from build123d import *

# Parameters (mm, degrees)
ESBO_O1_W                = 5
ESBO_O1_H                = 4.65
RESSALTO_EXTRUS_O1_DEPTH = 120
RESSALTO_EXTRUS_O2_DEPTH = 4.75
F_3_0MM_DOWEL_HOLE3_D    = 3
CUT_EXTRUDE2_DEPTH       = 10
FILLET4_START            = -3
FILLET4_DEPTH            = 6
FILLET1_SIZE             = 0.5
FILLET6_START            = -2.325
FILLET6_DEPTH            = 4.65
FILLET7_START            = -2.325
FILLET7_DEPTH            = 4.65


with BuildPart() as part:
    # Esboço1 → Ressalto-extrusão1 (new body)
    with BuildSketch(Plane(origin=(0, 0, 0), x_dir=(0, 0, -1), z_dir=(1, 0, 0))):
        with Locations((-2.5, 0)):
            Rectangle(ESBO_O1_W, ESBO_O1_H)
    extrude(amount=RESSALTO_EXTRUS_O1_DEPTH)

    # Esboço2 → Ressalto-extrusão2 (add)
    with BuildSketch(Plane(origin=(0, 2.325, 0), x_dir=(1, 0, 0), z_dir=(0, 1, 0))):
        Polygon((75, 0), (87.5, 0), (86.75, 4.5), align=None)
    extrude(amount=-RESSALTO_EXTRUS_O2_DEPTH)

    # Ø3.0mm Dowel Hole3 (through all)
    with Locations(Plane(origin=(0, 0, 0), x_dir=(-1, 0, 0), z_dir=(0, 0, -1))):
        with Locations((-5, 0), (-10, 0), (-15, 0), (-20, 0)):
            Hole(F_3_0MM_DOWEL_HOLE3_D / 2)

    # Sketch12 → Cut-Extrude2 (cut)
    with BuildSketch(Plane(origin=(0, 2.325, 0), x_dir=(1, 0, 0), z_dir=(0, 1, 0))):
        with BuildLine():
            Line((120, -2.5), (108.780523662, -2.5))
            ThreePointArc((108.780523662, -2.5), (105.971779801, -1.840547319), (103.75, 0))
            Line((103.75, 0), (120, 0))
            Line((120, 0), (120, -2.5))
        make_face()
    extrude(amount=-CUT_EXTRUDE2_DEPTH, mode=Mode.SUBTRACT)

    # Fillet4: read off the stored shape, not the designer's step
    # Fillet4 outline → Fillet4 (cut)
    with BuildSketch(Plane(origin=(0, 0, 0), x_dir=(1, 0, 0), z_dir=(0, 1, 0)).offset(FILLET4_START)):
        with BuildLine():
            add(Edge.make_bspline(
                [(104.477311177, -0.805478659), (103.613151376, 0), (102.431809752, 0)],
                knots=[0, 0, 0, 1, 1, 1], degree=2, weights=[1, 2.791376365, 1]))
            ThreePointArc((104.477311177, -0.805478659), (104.096310112, -0.418401518), (103.75, 0))
            Line((103.75, 0), (102.431809752, 0))
        make_face()
        with BuildLine():
            Line((120, -2.5), (117.041960108, -2.5))
            add(Edge.make_bspline(
                [(120, -5), (119.577422873, -2.5), (117.041960108, -2.5)],
                knots=[0, 0, 0, 1, 1, 1], degree=2, weights=[1, 2.291287847, 1]))
            Line((120, -5), (120, -2.5))
        make_face()
    extrude(amount=FILLET4_DEPTH, mode=Mode.SUBTRACT)

    # Fillet1
    # a fillet whose section is not a circle: 0.5 mm, written as the material it takes off along each edge
    with BuildSketch(Plane(origin=(20, 0, 0), x_dir=(1, 0, 0), z_dir=(0, -1, 0))) as fillet1_piece_1:
        with BuildLine():
            Bezier((1.5 + FILLET1_SIZE, 0), (1.5, 0), (1.5, FILLET1_SIZE), weights=[1, 0.353553391, 1])
            Line((1.5, FILLET1_SIZE), (1.5 - FILLET1_SIZE * 0.02, FILLET1_SIZE))
            Line((1.5 - FILLET1_SIZE * 0.02, FILLET1_SIZE), (1.5 - FILLET1_SIZE * 0.02, -FILLET1_SIZE * 0.02))
            Line((1.5 - FILLET1_SIZE * 0.02, -FILLET1_SIZE * 0.02), (1.5 + FILLET1_SIZE, -FILLET1_SIZE * 0.02))
            Line((1.5 + FILLET1_SIZE, -FILLET1_SIZE * 0.02), (1.5 + FILLET1_SIZE, 0))
        make_face()
    revolve(axis=Axis((20, 0, 0), (0, 0, 1)), mode=Mode.SUBTRACT)
    with BuildSketch(Plane(origin=(15, 0, 0), x_dir=(1, 0, 0), z_dir=(0, -1, 0))) as fillet1_piece_2:
        with BuildLine():
            Bezier((1.5 + FILLET1_SIZE, 0), (1.5, 0), (1.5, FILLET1_SIZE), weights=[1, 0.353553391, 1])
            Line((1.5, FILLET1_SIZE), (1.5 - FILLET1_SIZE * 0.02, FILLET1_SIZE))
            Line((1.5 - FILLET1_SIZE * 0.02, FILLET1_SIZE), (1.5 - FILLET1_SIZE * 0.02, -FILLET1_SIZE * 0.02))
            Line((1.5 - FILLET1_SIZE * 0.02, -FILLET1_SIZE * 0.02), (1.5 + FILLET1_SIZE, -FILLET1_SIZE * 0.02))
            Line((1.5 + FILLET1_SIZE, -FILLET1_SIZE * 0.02), (1.5 + FILLET1_SIZE, 0))
        make_face()
    revolve(axis=Axis((15, 0, 0), (0, 0, 1)), mode=Mode.SUBTRACT)
    with BuildSketch(Plane(origin=(10, 0, 0), x_dir=(1, 0, 0), z_dir=(0, -1, 0))) as fillet1_piece_3:
        with BuildLine():
            Bezier((1.5 + FILLET1_SIZE, 0), (1.5, 0), (1.5, FILLET1_SIZE), weights=[1, 0.353553391, 1])
            Line((1.5, FILLET1_SIZE), (1.5 - FILLET1_SIZE * 0.02, FILLET1_SIZE))
            Line((1.5 - FILLET1_SIZE * 0.02, FILLET1_SIZE), (1.5 - FILLET1_SIZE * 0.02, -FILLET1_SIZE * 0.02))
            Line((1.5 - FILLET1_SIZE * 0.02, -FILLET1_SIZE * 0.02), (1.5 + FILLET1_SIZE, -FILLET1_SIZE * 0.02))
            Line((1.5 + FILLET1_SIZE, -FILLET1_SIZE * 0.02), (1.5 + FILLET1_SIZE, 0))
        make_face()
    revolve(axis=Axis((10, 0, 0), (0, 0, 1)), mode=Mode.SUBTRACT)
    with BuildSketch(Plane(origin=(5, 0, 0), x_dir=(1, 0, 0), z_dir=(0, -1, 0))) as fillet1_piece_4:
        with BuildLine():
            Bezier((1.5 + FILLET1_SIZE, 0), (1.5, 0), (1.5, FILLET1_SIZE), weights=[1, 0.353553391, 1])
            Line((1.5, FILLET1_SIZE), (1.5 - FILLET1_SIZE * 0.02, FILLET1_SIZE))
            Line((1.5 - FILLET1_SIZE * 0.02, FILLET1_SIZE), (1.5 - FILLET1_SIZE * 0.02, -FILLET1_SIZE * 0.02))
            Line((1.5 - FILLET1_SIZE * 0.02, -FILLET1_SIZE * 0.02), (1.5 + FILLET1_SIZE, -FILLET1_SIZE * 0.02))
            Line((1.5 + FILLET1_SIZE, -FILLET1_SIZE * 0.02), (1.5 + FILLET1_SIZE, 0))
        make_face()
    revolve(axis=Axis((5, 0, 0), (0, 0, 1)), mode=Mode.SUBTRACT)

    # Fillet5
    # a fillet whose section is not a circle: 2 mm, written as the material it takes off along each edge
    with BuildSketch(Plane(origin=(86.75, 8.443980956, -4.5), x_dir=(-0.9338567516961642, 0, 0.35764726660704255), z_dir=(0, -1, 0))) as fillet5_piece_1:
        with BuildLine():
            Bezier((2.447592383, 0), (0, 0), (0.487697434, -2.398511973), weights=[1, 1.265499122, 1])
            Line((0.487697434, -2.398511973), (0, 0))
            Line((0, 0), (2.447592383, 0))
        make_face()
    extrude(amount=16.987961913, mode=Mode.SUBTRACT)

    # Fillet6: read off the stored shape, not the designer's step
    # Fillet6 outline → Fillet6 (add)
    with BuildSketch(Plane(origin=(0, 0, 0), x_dir=(1, 0, 0), z_dir=(0, 1, 0)).offset(FILLET6_START)):
        with BuildLine():
            Line((75, 0), (75.345414741, 0.132286497))
            add(Edge.make_bspline(
                [(75.345414741, 0.132286497), (75, 0), (74.630120208, 0)],
                knots=[0, 0, 0, 1, 1, 1], degree=2, weights=[1, 1.966650326, 1]))
            Line((74.630120208, 0), (75, 0))
        make_face()
    extrude(amount=FILLET6_DEPTH)

    # Fillet7: read off the stored shape, not the designer's step
    # Fillet7 outline → Fillet7 (add)
    with BuildSketch(Plane(origin=(0, 0, 0), x_dir=(1, 0, 0), z_dir=(0, 1, 0)).offset(FILLET7_START)):
        with BuildLine():
            Line((87.5, 0), (89.194254177, 0))
            add(Edge.make_bspline(
                [(89.194254177, 0), (87.5, 0), (87.221466329, 1.671202025)],
                knots=[0, 0, 0, 1, 1, 1], degree=2, weights=[1, 1.526039965, 1]))
            Line((87.221466329, 1.671202025), (87.5, 0))
        make_face()
    extrude(amount=FILLET7_DEPTH)


solid = part.part
Can you work these out from the model? Positions are in its coordinate system, mm. A direction names the side the tool comes from. Coordinates: 2 decimals unless noted, no trailing zeros. Loops run counter-clockwise (first coordinate to the right, second up) from the corner with the lowest first, then second, coordinate; pieces in that order, holes last. Notation, with made-up numbers: M 87,56 L 112,56 A25 cw 112,91 Z; hole C 89,-29 d6. An arc over 180 degrees is marked long. Answer as CSV lines item,"result". Start each with the question number.
1. If I drill on probe 1 along X at (y, z) = (0.65, 4.25); probe 2 along X at (y, z) = (-0.55, 1.5); probe 3 along Y at (x, z) = (15, 1.45) (3 decimals), over which ranges is the centre line in solid material (lowest first)? Write a range as [from, to].
2. For pin 1 Ø1.5 at (y, z) = (0, 0) entering from +X; pin 2 Ø2.5 at (x, y) = (49, 0.5) entering from -Z; pin 3 Ø2.5 at (x, y) = (112, 0.5) entering from -Z, each with a flat end and sliding along its axis, tell me the tip position at first contact or that it passes through.
3. For faces 1 (the face through (96, 0, 0)), 2 (the face through (45, 0, 0)), 3 (the face through (83, -2.425, -2)), which set-ups out of +Z, -Z, +X, -X, +Y, -Y let a thin tool reach every point of the face, with its end or its side?
4. Thinking about a two-plate mould opening in Y: for faces 4 (the face through (59, 2.325, 2)), 5 (the face through (13.5, 0.07, 2.78)), 6 (the face through (0, 0, 3)), which applies, +Y half, -Y half, draft (parallel to the pull), parting line (faces both ways), or undercut?
5. Suppose I cut it at B-B, the plane x = 66. List the corners of the cut face in (y, z) for me (3 decimals).
6. Suppose I cut it at A-A, the plane y = 0. Count the separate pieces of the cut face and the enclosed holes in it, plus the area to 3 significant figures.
Output:
1,probe 1,"x = [0, 3.65], [6.35, 8.65], [11.35, 13.65], [16.35, 18.65], [21.35, 119.86]"
1,probe 2,"x = [0, 3.6], [6.4, 8.6], [11.4, 13.6], [16.4, 18.6], [21.4, 105.37]"
1,probe 3,"y = [-2.325, -1.5], [1.5, 2.325]"
2,pin 1,"stops at x = 104.42"
2,pin 2,"stops at z = 0"
2,pin 3,"stops at z = 2.5"
3,face 1,"-Z, +X, +Y, -Y"
3,face 2,"-Z, -X, +Y, -Y"
3,face 3,"+Z, -Z, +X, -X, -Y"
4,face 4,"+Y half"
4,face 5,"undercut"
4,face 6,"draft"
5,outline,"M -2.325,0 L 2.325,0 L 2.325,5 L -2.325,5 Z"
6,separate pieces,"5"
6,enclosed holes,"0"
6,area,"529 mm^2"
